Geometry: final body of the model. Coordinates: model frame, mm. Coordinates: 2 decimals unless noted, no trailing zeros. Loops run counter-clockwise (first coordinate to the right, second up) from the corner with the lowest first, then second, coordinate; pieces in that order, holes last. Notation, with made-up numbers: (-34.5, -40) - (17.5, -40) arc R35 cw to (17.5, -7) - close; hole circle Ø4 at (67, 63). An arc over 180 degrees is marked (long way). Put each result on its own line as item: value. Start each with the question number.
1) Material intervals for line 1 along Y through (x, z) = (-22.86, 6.75); line 2 along Y through (x, z) = (24, 10.75); line 3 along X through (y, z) = (59, 7.75), sorted ascending. Write a range as from..to.
2) Section C-C on z = 10. Count the separate pieces of the cut face and the enclosed holes in it, and give its area (3 significant figures).
3) Contact query for flat-ended pins moving along their axis: pin 1 Ø1 at (y, z) = (-28.5, 4) entering from -X; pin 2 Ø2.5 at (x, y) = (-22.86, 38.735) entering from +Z. Output: stop coordinate, or through.
4) Section A-A on x = -22.86. Output: boundary loops of the cut face in (y, z), and give its area (3 significant figures).
5) Draft query along Y for faces 1 (the cylindrical face through (-21.394, -39.343, 6.439)), 2 (the cylindrical face through (-48.89, 80.74, 6.33)), 3 (the cylindrical face through (24.326, -39.343, 6.439)), 4 (the cylindrical face through (-49.351, -1.067, 11.172)). Return one class per face: +Y half, -Y half, draft (parallel to the pull), parting line (faces both ways), or undercut.
6) Section B-B on y = 42. Output: boundary loops of the cut face in (x, z).
```python
from build123d import *

# Parameters (mm, degrees)
F1_DEPTH = 12.7
F2_R     = 5.08
F3_R     = 1.5875
F4_DEPTH = 12.701


with BuildPart() as f1:
    # F0 (on Top) → F1 (new body)
    with BuildSketch(Plane.XY):
        with BuildLine():
            ThreePointArc((50.8, 76.2), (48.940128, 80.690128), (44.45, 82.55))
            Line((44.45, 82.55), (-44.45, 82.55))
            ThreePointArc((-44.45, 82.55), (-48.940128, 80.690128), (-50.8, 76.2))
            Line((-50.8, 76.2), (-50.8, -76.2))
            ThreePointArc((-50.8, -76.2), (-48.940128, -80.690128), (-44.45, -82.55))
            Line((-44.45, -82.55), (44.45, -82.55))
            ThreePointArc((44.45, -82.55), (48.940128, -80.690128), (50.8, -76.2))
            Line((50.8, -76.2), (50.8, 76.2))
        make_face()
    extrude(amount=F1_DEPTH)

    # F2
    f2_edges = [f1.edges().sort_by_distance(p)[0] for p in [
        (48.940128, 80.690128, 12.7),
        (0, 82.55, 12.7),
        (-48.940128, 80.690128, 12.7),
        (-50.8, 0, 12.7),
        (-48.940128, -80.690128, 12.7),
        (0, -82.55, 12.7),
        (48.940128, -80.690128, 12.7),
        (50.8, 0, 12.7),
        (48.940128, 80.690128, 0),
        (0, 82.55, 0),
        (-48.940128, 80.690128, 0),
        (-50.8, 0, 0),
        (-48.940128, -80.690128, 0),
        (0, -82.55, 0),
        (48.940128, -80.690128, 0),
        (50.8, 0, 0),
    ]]
    fillet(f2_edges, radius=F2_R)

    # F3 (on face) → F4 (cut, through all)
    with BuildSketch(Plane.XY.offset(12.7)):
        with Locations((-22.86, 38.735)):
            Circle(F3_R)
        with Locations((22.86, 38.735)):
            Circle(F3_R)
        with Locations((-22.86, -38.735)):
            Circle(F3_R)
        with Locations((22.86, -38.735)):
            Circle(F3_R)
    extrude(amount=-F4_DEPTH, mode=Mode.SUBTRACT)


solid = f1.part
```
Answer block:
1. line 1: y = -82.55..-40.32, -37.15..37.15, 40.32..82.55
1. line 2: y = -81.47..-39.84, -37.63..37.63, 39.84..81.47
1. line 3: x = -50.8..50.8
2. separate pieces: 1
2. enclosed holes: 4
2. area: 16,400 mm²
3. pin 1: stops at x = -50.77
3. pin 2: passes through
4. outline: (-82.55, 5.08) arc R5.08 ccw to (-77.47, 0) - (-40.32, 0) - (-40.32, 12.7) - (-77.47, 12.7) arc R5.08 ccw to (-82.55, 7.62) - close; (-37.15, 0) - (37.15, 0) - (37.15, 12.7) - (-37.15, 12.7) - close; (40.32, 0) - (77.47, 0) arc R5.08 ccw to (82.55, 5.08) - (82.55, 7.62) arc R5.08 ccw to (77.47, 12.7) - (40.32, 12.7) - close
4. area: 1,990 mm²
5. face 1: undercut
5. face 2: +Y half
5. face 3: undercut
5. face 4: draft
6. outline: (-50.8, 5.08) arc R5.08 ccw to (-45.72, 0) - (45.72, 0) arc R5.08 ccw to (50.8, 5.08) - (50.8, 7.62) arc R5.08 ccw to (45.72, 12.7) - (-45.72, 12.7) arc R5.08 ccw to (-50.8, 7.62) - close
